Geometry: final body of the model. Coordinates: model frame, mm. A direction names the side the tool comes from. Give positions to 0.01 mm unless a question says otherwise; leave off trailing zeros. Loops run counter-clockwise (first coordinate to the right, second up) from the corner with the lowest first, then second, coordinate; pieces in that order, holes last. Notation, with made-up numbers: (27.25, -21.5) -> (53.25, -21.5) arc R32 ccw to (53.25, 9.5) -> close; hole circle Ø2 at (-32.5, 73.5). An arc over 180 degrees is marked (long way). Answer in a Markdown table with one row per item. Add a question column.
1) First-contact query: P1, Ø6, axis at x = -4, z = -1, coming from the +Y side (3 decimals); P2, Ø2.5, axis at x = 0, y = 0, coming from the -Z side; P3, Ø3, axis at y = -5, z = 11, coming from the +X side. Flat tips, straight axial feed; report the tip coordinate or a pass-through.
2) Line query: line 1 (X direction, y = 0, z = -9); line 2 (Y direction, x = 0, z = -8.5) (3 decimals); line 3 (X direction, y = -0.75, z = 10.5). Output: solid intervals per line, ascending. Write a range as from..to.
3) Access query for faces 4 (the flat face through (-6, -3, 18.612)), 5 (the flat face through (6, -3, 18.612)), 6 (the flat face through (-6, 3, 18.612)), 7 (the flat face through (0, 6.5, 18.612)), 8 (the flat face through (6, 3, 18.612)). Directions: +Z, -Z, +X, -X, +Y, -Y. A direction counts if a zero-diameter tool reaches every point of the face in a straight line with its end or side. Return the directions, or none.
4) Draft query along Y for faces 1 (the cylindrical face through (-5.948, 3.448, -3.653)), 2 (the cylindrical face through (-1.38, -6.2, 22.64)), 3 (the cylindrical face through (1.926, 0.607, -0.372)). Return one class per face: +Y half, -Y half, draft (parallel to the pull), parting line (faces both ways), or undercut.
5) Section query C-C (y = 0.75). Return the cut outline in (x, z).
6) Section query D-D (y = 3.25). Return the cut outline in (x, z).
7) Section query A-A (z = 5.5). Return the cut outline in (x, y) (3 decimals), plus the area to 3 significant figures.
```python
from build123d import *

# Parameters (mm, degrees)
SKETCH1_R                            = 2.0193
BOSS_EXTRUDE1_DEPTH                  = 26.549999986
F_10_32_TAPPED_HOLE1_D               = 4.0386
F_10_32_TAPPED_HOLE1_DEPTH           = 12.02944
F_10_32_TAPPED_HOLE1_TIP             = 1.213317848
F_10_32_TAPPED_HOLE1_ON_FACE_2_D     = 4.0386
F_10_32_TAPPED_HOLE1_ON_FACE_2_DEPTH = 12.02944
F_10_32_TAPPED_HOLE1_ON_FACE_2_TIP   = 1.213317848
SKETCH5_R                            = 6.874999966
SKETCH5_R_2                          = 6.35
CUT_EXTRUDE1_DEPTH                   = 7.9375


with BuildPart() as part:
    # Sketch1 → Boss-Extrude1 (new, symmetric)
    with BuildSketch(Plane.XY):
        with BuildLine():
            ThreePointArc((0.893039571, 6.816751782), (0, 6.874999966), (-0.893039571, 6.816751782))
            Line((-0.893039571, 6.816751782), (-5.456960429, 4.181770846))
            ThreePointArc((-5.456960429, 4.181770846), (-5.953924622, 3.437499983), (-6.35, 2.634980936))
            Line((-6.35, 2.634980936), (-6.35, -2.634980936))
            ThreePointArc((-6.35, -2.634980936), (-5.953924622, -3.437499983), (-5.456960429, -4.181770846))
            Line((-5.456960429, -4.181770846), (-0.893039571, -6.816751782))
            ThreePointArc((-0.893039571, -6.816751782), (0, -6.874999966), (0.893039571, -6.816751782))
            Line((0.893039571, -6.816751782), (5.456960429, -4.181770846))
            ThreePointArc((5.456960429, -4.181770846), (5.953924622, -3.437499983), (6.35, -2.634980936))
            Line((6.35, -2.634980936), (6.35, 2.634980936))
            ThreePointArc((6.35, 2.634980936), (5.953924622, 3.437499983), (5.456960429, 4.181770846))
            Line((5.456960429, 4.181770846), (0.893039571, 6.816751782))
        make_face()
        Circle(SKETCH1_R, mode=Mode.SUBTRACT)
    extrude(amount=BOSS_EXTRUDE1_DEPTH, both=True)

    # #10-32 Tapped Hole1
    with Locations(Plane.XY.offset(26.549999986)):
        with Locations((0, 0)):
            Hole(F_10_32_TAPPED_HOLE1_D / 2, depth=F_10_32_TAPPED_HOLE1_DEPTH)
            with Locations((0, 0, -(F_10_32_TAPPED_HOLE1_DEPTH + F_10_32_TAPPED_HOLE1_TIP / 2))):  # 118° drill point
                Cone(0, F_10_32_TAPPED_HOLE1_D / 2, F_10_32_TAPPED_HOLE1_TIP, mode=Mode.SUBTRACT)

    # #10-32 Tapped Hole1 on face 2
    with Locations(Plane.XY.offset(-26.549999986)):
        with Locations((0, 0)):
            Hole(F_10_32_TAPPED_HOLE1_ON_FACE_2_D / 2, depth=F_10_32_TAPPED_HOLE1_ON_FACE_2_DEPTH)
            with Locations((0, 0, -(F_10_32_TAPPED_HOLE1_ON_FACE_2_DEPTH + F_10_32_TAPPED_HOLE1_ON_FACE_2_TIP / 2))):  # 118° drill point
                Cone(0, F_10_32_TAPPED_HOLE1_ON_FACE_2_D / 2, F_10_32_TAPPED_HOLE1_ON_FACE_2_TIP, mode=Mode.SUBTRACT)

    # Sketch5 → Cut-Extrude1 (cut)
    with BuildSketch(Plane.XY.offset(26.549999986)):
        Circle(SKETCH5_R)
        Circle(SKETCH5_R_2, mode=Mode.SUBTRACT)
    extrude(amount=-CUT_EXTRUDE1_DEPTH, mode=Mode.SUBTRACT)


solid = part.part
```
Evaluation:
| question | item | result |
|---|---|---|
| 1 | P1 | y = 6.755 |
| 1 | P2 | through |
| 1 | P3 | x = 5.92 |
| 2 | line 1 | -6.35..-2.02, 2.02..6.35 |
| 2 | line 2 | -6.875..-2.019, 2.019..6.875 |
| 2 | line 3 | -6.35..-1.87, 1.87..6.35 |
| 3 | face 4 | +Z, -X, -Y |
| 3 | face 5 | +Z, +X, -Y |
| 3 | face 6 | +Z, -X, +Y |
| 3 | face 7 | +Z, +Y |
| 3 | face 8 | +Z, +X, +Y |
| 4 | face 1 | +Y half |
| 4 | face 2 | parting line |
| 4 | face 3 | undercut |
| 5 | outline | (-6.35, -26.55) -> (-1.87, -26.55) -> (-1.87, 26.55) -> (-6.31, 26.55) -> (-6.31, 18.61) -> (-6.35, 18.61) -> close; (1.87, -26.55) -> (6.35, -26.55) -> (6.35, 18.61) -> (6.31, 18.61) -> (6.31, 26.55) -> (1.87, 26.55) -> close |
| 6 | outline | (-6.06, -26.55) -> (6.06, -26.55) -> (6.06, 18.61) -> (5.46, 18.61) -> (5.46, 26.55) -> (-5.46, 26.55) -> (-5.46, 18.61) -> (-6.06, 18.61) -> close |
| 7 | outline | (-6.35, -2.635) arc R6.875 ccw to (-5.457, -4.182) -> (-0.893, -6.817) arc R6.875 ccw to (0.893, -6.817) -> (5.457, -4.182) arc R6.875 ccw to (6.35, -2.635) -> (6.35, 2.635) arc R6.875 ccw to (5.457, 4.182) -> (0.893, 6.817) arc R6.875 ccw to (-0.893, 6.817) -> (-5.457, 4.182) arc R6.875 ccw to (-6.35, 2.635) -> close; hole circle Ø4.039 at (0, 0) |
| 7 | area | 125 mm² |
